The listing builds one solid part. Answer for the finished solid, in the listing's coordinates (mm). Face numbers are marked on the shaded views. Coordinates: 2 decimals unless noted, no trailing zeros. Write each loop counter-clockwise with the first axis right and the second up, starting at its lowest first coordinate (ties: lowest second). Pieces come first, ordered by that corner, then holes.
```python
from build123d import *

# Parameters (mm, degrees)
F0_W     = 52.6
F0_H     = 28.8
F0_W_2   = 49.6
F0_H_2   = 25.8
F0_W_3   = 46.6
F0_H_3   = 22.8
F0_W_4   = 2
F0_H_4   = 20
F1_DEPTH = 1.5
F2_R     = 3
F3_DEPTH = 1.8
F4_R     = 2
F5_R     = 1.3


with BuildPart() as f1:
    # F0 (on Top) → F1 (new body)
    with BuildSketch(Plane.XY):
        with Locations((3.602296, 3.818181)):
            Rectangle(F0_W, F0_H)
        with Locations((3.602296, 3.818181)):
            Rectangle(F0_W_2, F0_H_2, mode=Mode.SUBTRACT)
        with Locations((3.602296, 3.818181)):
            Rectangle(F0_W_2, F0_H_2)
        with Locations((3.602296, 3.818181)):
            Rectangle(F0_W_3, F0_H_3, mode=Mode.SUBTRACT)
        with Locations((3.602296, 3.818181)):
            Rectangle(F0_W_3, F0_H_3)
        with Locations((-16.697704, 3.818181)):
            Rectangle(F0_W_4, F0_H_4, mode=Mode.SUBTRACT)
        with Locations((-13.097704, 3.818181)):
            Rectangle(F0_W_4, F0_H_4, mode=Mode.SUBTRACT)
        with Locations((-9.497704, 3.818181)):
            Rectangle(F0_W_4, F0_H_4, mode=Mode.SUBTRACT)
        with Locations((-5.897704, 3.818181)):
            Rectangle(F0_W_4, F0_H_4, mode=Mode.SUBTRACT)
        with Locations((-2.297704, 3.818181)):
            Rectangle(F0_W_4, F0_H_4, mode=Mode.SUBTRACT)
    extrude(amount=-F1_DEPTH)

    # F2
    f2_edges = [f1.edges().sort_by_distance(p)[0] for p in [
        (-22.697704, 18.218181, -0.75),
        (29.902296, 18.218181, -0.75),
        (29.902296, -10.581819, -0.75),
        (-22.697704, -10.581819, -0.75),
    ]]
    fillet(f2_edges, radius=F2_R)

    # F0 (on Top) → F3 (join)
    with BuildSketch(Plane.XY):
        with Locations((3.602296, 3.818181)):
            Rectangle(F0_W_2, F0_H_2)
        with Locations((3.602296, 3.818181)):
            Rectangle(F0_W_3, F0_H_3, mode=Mode.SUBTRACT)
    extrude(amount=F3_DEPTH)

    # F4
    f4_edges = [f1.edges().sort_by_distance(p)[0] for p in [
        (-21.197704, -9.081819, 0.9),
        (-21.197704, 16.718181, 0.9),
        (28.402296, 16.718181, 0.9),
        (28.402296, -9.081819, 0.9),
    ]]
    fillet(f4_edges, radius=F4_R)

    # F5
    f5_edges = [f1.edges().sort_by_distance(p)[0] for p in [
        (-19.697704, 15.218181, 0.9),
        (-19.697704, -7.581819, 0.9),
        (26.902296, -7.581819, 0.9),
        (26.902296, 15.218181, 0.9),
    ]]
    fillet(f5_edges, radius=F5_R)


solid = f1.part
```
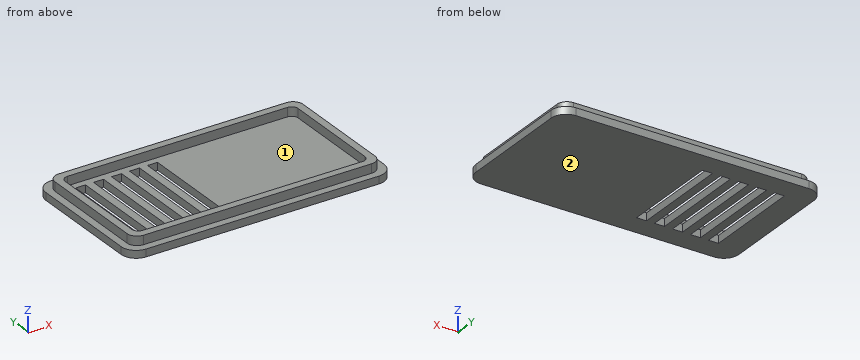
(1) Section D-D, the plane y = 16 is taken. Write down the section's boundary in (x, z).
(2) Find the intervals of material crossed by probe 1 along X at (y, z) = (12.25, -1.4); probe 2 along Y at (x, z) = (20.5, 1.3); probe 3 along X at (y, z) = (11, 0.1), in increasing order.
(3) Section B-B, the plane z = 0.7 is taken. Write down the section's boundary in (x, y), plus the area to 3 significant figures.
(4) Section A-A, the plane y = -0.75 is taken. State how many separate pieces and enclosed holes the cut face has, plus the area to 3 significant figures.
(5) Section C-C, the plane x = 14 is taken. Write down the section's boundary in (y, z).
(6) Each of these flat-tipped pins is pushed along its axis until it touches: pin 1 (0.5 mm diameter, centred on x = 2, z = 1, fed in from +Y); pin 2 (1.5 mm diameter, centred on x = 24, y = 13.5, fed in from +Z); pin 3 (0.9 mm diameter, centred on y = 9, z = 1, fed in from -X). Where does it stop, or does it pass through?
(7) For a pull along X with two mould halves and no side action, classify the marked faces 1 and 2 as pulls with the +X half, pulls with the -X half, needs draft (parallel to the pull), parting line crosses it, or undercut.
Solution:
1. outline: (-22.59, -1.5) - (29.8, -1.5) - (29.8, 0) - (27.94, 0) - (27.94, 1.8) - (-20.73, 1.8) - (-20.73, 0) - (-22.59, 0) - close
2. probe 1: x = -22.7 to -17.7, -15.7 to -14.1, -12.1 to -10.5, -8.5 to -6.9, -4.9 to -3.3, -1.3 to 29.9
2. probe 2: y = -9.08 to -7.58, 15.22 to 16.72
2. probe 3: x = -21.2 to -19.7, 26.9 to 28.4
3. outline: (-21.2, -7.08) arc R2 ccw to (-19.2, -9.08) - (26.4, -9.08) arc R2 ccw to (28.4, -7.08) - (28.4, 14.72) arc R2 ccw to (26.4, 16.72) - (-19.2, 16.72) arc R2 ccw to (-21.2, 14.72) - close; hole (-19.7, -6.28) arc R1.3 ccw to (-18.4, -7.58) - (25.6, -7.58) arc R1.3 ccw to (26.9, -6.28) - (26.9, 13.92) arc R1.3 ccw to (25.6, 15.22) - (-18.4, 15.22) arc R1.3 ccw to (-19.7, 13.92) - close
3. area: 215 mm2
4. separate pieces: 6
4. enclosed holes: 0
4. area: 69.3 mm2
5. outline: (-10.58, -1.5) - (18.22, -1.5) - (18.22, 0) - (16.72, 0) - (16.72, 1.8) - (15.22, 1.8) - (15.22, 0) - (-7.58, 0) - (-7.58, 1.8) - (-9.08, 1.8) - (-9.08, 0) - (-10.58, 0) - close
6. pin 1: stops at y = 16.72
6. pin 2: stops at z = 0
6. pin 3: stops at x = -21.2
7. face 1: undercut
7. face 2: needs draft
